from build123d import *

# Parameters (mm, degrees)
SKETCH_1_W      = 33
SKETCH_1_H      = 28
EXTRUDE_1_DEPTH = 2
SKETCH_2_W      = 32
SKETCH_2_H      = 27
SKETCH_2_W_2    = 29
SKETCH_2_H_2    = 24
EXTRUDE_2_DEPTH = 4


with BuildPart() as part:
    # 草图1 → 凸台-拉伸1 (new body)
    with BuildSketch(Plane(origin=(0, 0, 0), x_dir=(1, 0, 0), z_dir=(0, 1, 0))):
        with Locations((16.5, -14)):
            Rectangle(SKETCH_1_W, SKETCH_1_H)
    extrude(amount=EXTRUDE_1_DEPTH)

    # 草图2 → 凸台-拉伸2 (add)
    with BuildSketch(Plane(origin=(0, 2, 0), x_dir=(1, 0, 0), z_dir=(0, 1, 0))):
        with Locations((16.5, -14)):
            Rectangle(SKETCH_2_W, SKETCH_2_H)
        with Locations((16.5, -14)):
            Rectangle(SKETCH_2_W_2, SKETCH_2_H_2, mode=Mode.SUBTRACT)
    extrude(amount=EXTRUDE_2_DEPTH)


solid = part.part
CAD build for the part. Positions are in the model's coordinates, mm. A direction names the side the tool comes from. Round coordinates to 2 decimals unless told otherwise and drop trailing zeros. Write each loop counter-clockwise with the first axis right and the second up, starting at its lowest first coordinate (ties: lowest second). Pieces come first, ordered by that corner, then holes. Notation, with made-up numbers: M 61.25,38.5 L 103.25,38.5 A22 cw 103.25,55.5 Z; hole C -2,-34.75 d7. An arc over 180 degrees is marked long. Put each result on its own line as item: value. Start each with the question number.
1) Pin check, flat tips, straight feed: pin 1 Ø8 at (x, z) = (7, 14) entering from +Y; pin 2 Ø3 at (y, z) = (4, 16.5) entering from -X; pin 3 Ø1.2 at (x, y) = (13.5, 4) entering from +Z. Stop position of each tip, or through.
2) Drill centre lines: probe 1 along X at (y, z) = (3, 21.75); probe 2 along Z at (x, y) = (9, 2.35); probe 3 along Y at (x, z) = (20.5, 16.5). Where is each one in solid material? Low to high. Write a range as [from, to].
3) Saw through at C-C, the plane z = 16.5. Write the cut outline in (x, y).
4) 3-axis set-ups, long thin cutter, end or side, ignore diameter. For faces 1 (the flat face through (16, 4, 2)), 2 (the flat face through (16, 4, 0.5)), 3 (the flat face through (32.5, 4, 14)): which of +Z, -Z, +X, -X, +Y, -Y reach the whole face in a straight line?
5) Pull direction X, two halves, no side cores. Call faces 4 (the flat face through (2, 4, 14)), 5 (the flat face through (0, 1, 14)), 6 (the flat face through (16, 1, 28)): pulls with the +X half, pulls with the -X half, needs draft (parallel to the pull), parting line crosses it, or undercut.
6) Saw through at B-B, the plane y = 3. Write the cut outline in (x, z), and give its area (3 significant figures).
7) Saw through at A-A, the plane x = 4. Write the cut outline in (y, z), and give its area (3 significant figures).
Resolved:
1. pin 1: y = 2
1. pin 2: x = 0.5
1. pin 3: z = 27.5
2. probe 1: [0.5, 2], [31, 32.5]
2. probe 2: [0.5, 2], [26, 27.5]
2. probe 3: [0, 2]
3. outline: M 0,0 L 33,0 L 33,2 L 32.5,2 L 32.5,6 L 31,6 L 31,2 L 2,2 L 2,6 L 0.5,6 L 0.5,2 L 0,2 Z
4. face 1: +Y
4. face 2: -Z, +X, -X, +Y
4. face 3: +Z, -Z, +X, +Y
5. face 4: undercut
5. face 5: pulls with the -X half
5. face 6: needs draft
6. outline: M 0.5,0.5 L 32.5,0.5 L 32.5,27.5 L 0.5,27.5 Z; hole M 2,2 L 31,2 L 31,26 L 2,26 Z
6. area: 168 mm²
7. outline: M 0,0 L 2,0 L 2,0.5 L 6,0.5 L 6,2 L 2,2 L 2,26 L 6,26 L 6,27.5 L 2,27.5 L 2,28 L 0,28 Z
7. area: 68.0 mm²
